The model under review builds one solid part; all positions refer to its coordinate system, in mm. Round coordinates to 2 decimals unless told otherwise and drop trailing zeros. Order: outer loops, then holes, each group sorted by start corner. A loop starts at its lowest first (then second) coordinate and runs counter-clockwise, first axis right, second up.
```python
from build123d import *

# Parameters (mm, degrees)
SM_BASE_FLANGE_1_DEPTH = 105
FILLET_1_R             = 20


# Sheet-metal steps are written as plain solids
with BuildPart() as part:
    # Sketch 1 → 基体-法兰1 (new, symmetric)
    with BuildSketch(Plane.XY):
        with BuildLine():
            ThreePointArc((-50, -976.220390076), (0, -977.5), (50, -976.220390076))
            Line((50, -976.220390076), (50.613810742, -988.20468131))
            ThreePointArc((50.613810742, -988.20468131), (0, -989.5), (-50.613810742, -988.20468131))
            Line((-50.613810742, -988.20468131), (-50, -976.220390076))
        make_face()
    extrude(amount=SM_BASE_FLANGE_1_DEPTH, both=True)

    # 圆角1
    fillet_1_edges = [part.edges().sort_by_distance(p)[0] for p in [
        (-50.306905371, -982.212535693, 105),
        (-50.306905371, -982.212535693, -105),
        (50.306905371, -982.212535693, -105),
        (50.306905371, -982.212535693, 105),
    ]]
    fillet(fillet_1_edges, radius=FILLET_1_R)


solid = part.part
```
(1) Consider section A-A (x = -22.5). Write out the cut boundary in (y, z).
Data:
outline: (-989.24, -105) - (-977.24, -105) - (-977.24, 105) - (-989.24, 105) - close
(2) Consider section B-B (z = 6.5). Write out the cut boundary in (x, y), and give its area (3 significant figures).
Data:
outline: (-50.61, -988.2) arc R989.5 ccw to (50.61, -988.2) - (50, -976.22) arc R977.5 cw to (-50, -976.22) - close
area: 1,210 mm2
(3) To check wall thickness, follow probe 1 along X at (y, z) = (-987.75, -42); probe 2 along Y at (x, z) = (7, -83); probe 3 along Y at (x, z) = (29.5, -95.5). State the ranges of each line that lie inside material, in increasing order.
Data:
probe 1: x = -50.59 to 50.59
probe 2: y = -989.48 to -977.47
probe 3: y = -989.06 to -977.05
(4) Draft analysis for pull direction X (two halves, no side actions). For faces 1 (the cylindrical face through (-0.7, -977.5, 1.5)), 2 (the cylindrical face through (44.3, -982.503, 99.297)), 3 (the flat face through (0, -983, -105)), state which applies: pulls with the +X half, pulls with the -X half, needs draft (parallel to the pull), parting line crosses it, or undercut.
Data:
face 1: undercut
face 2: pulls with the +X half
face 3: needs draft
(5) Insertion check: pin 1 (3 mm diameter, centred on x = 9, z = -16, fed in from -Y); pin 2 (2 mm diameter, centred on x = 39, z = -51, fed in from -Y); pin 3 (3 mm diameter, centred on y = -985, z = -33, fed in from +X); pin 4 (2 mm diameter, centred on y = -987.5, z = 48, fed in from -X). Each pin has a flat end and moves straight along its axis. Give the tip position at first contact, or say it passes through.
Data:
pin 1: stops at y = -989.47
pin 2: stops at y = -988.77
pin 3: stops at x = 50.53
pin 4: stops at x = -50.61
